```python
from build123d import *

# Parameters (mm, degrees)
BOSS_EXTRUDE1_DEPTH          = 21.6
SKETCH3_OUTSIDE_W            = 131.808
SKETCH3_OUTSIDE_H            = 138.238
SKETCH3_OUTSIDE_R            = 20.784609691
CUT_EXTRUDE1_DEPTH           = 21.6
CUT_EXTRUDE1_DRAFT           = -60
M24_TAPPED_HOLE1_D           = 21
M24_TAPPED_HOLE1_CSINK_D     = 24.05
M24_TAPPED_HOLE1_CSINK_ANGLE = 90


with BuildPart() as part:
    # Sketch1 → Boss-Extrude1 (new body)
    with BuildSketch(Plane.XY):
        Polygon((20.784609691, -12), (20.784609691, 12), (0, 24), (-20.784609691, 12), (-20.784609691, -12), (0, -24), align=None)
    extrude(amount=BOSS_EXTRUDE1_DEPTH)


with BuildPart() as cut_extrude1_tool:
    # Sketch3 outside → Cut-Extrude1 (with draft: the straight prism first)
    with BuildSketch(Plane.XY.offset(21.6)):
        Rectangle(SKETCH3_OUTSIDE_W, SKETCH3_OUTSIDE_H)
        Circle(SKETCH3_OUTSIDE_R, mode=Mode.SUBTRACT)
    extrude(amount=-CUT_EXTRUDE1_DEPTH)
    # Cut-Extrude1: the draft: its side faces are tilted about the plane it starts from
    cut_extrude1_sides = [cut_extrude1_tool.faces().sort_by_distance(p)[0] for p in [
        (0, -69.119, 10.8),
        (65.904, 0, 10.8),
        (0, 69.119, 10.8),
        (-65.904, 0, 10.8),
        (-20.784609691, 0, 10.8),
    ]]
    draft(cut_extrude1_sides, Plane.XY.offset(21.6), CUT_EXTRUDE1_DRAFT)


with BuildPart() as part_1:
    add(part.part)

    # Cut-Extrude1: cut by cut_extrude1_tool
    add(cut_extrude1_tool.part, mode=Mode.SUBTRACT)

    # M24 Tapped Hole1 (through all)
    with Locations(Plane.XY.offset(21.6)):
        with Locations((0, 0)):
            CounterSinkHole(M24_TAPPED_HOLE1_D / 2, M24_TAPPED_HOLE1_CSINK_D / 2, counter_sink_angle=M24_TAPPED_HOLE1_CSINK_ANGLE)


solid = part_1.part
```
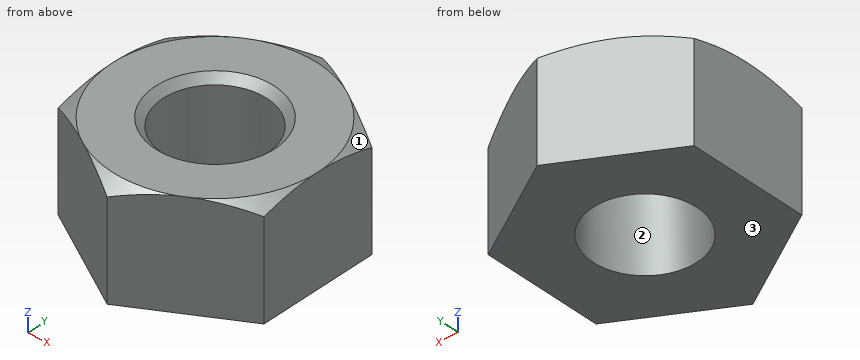
Here's how the part is built. I have some questions about the finished solid (model axes, mm). Face numbers are marked on the shaded views. Give positions to 0.01 mm unless a question says otherwise; leave off trailing zeros. Order: outer loops, then holes, each group sorted by start corner. A loop starts at its lowest first (then second) coordinate and runs counter-clockwise, first axis right, second up. Notation, with made-up numbers: (13.5, 17.5) - (28.5, 17.5) arc R14 ccw to (28.5, 31.5) - close; hole circle Ø8 at (53.5, 51.5). An arc over 180 degrees is marked (long way). Answer as a JSON object with one key per item and string values. Group by question number.
Item 1: If we section it at A-A on z = 2.5: Please give me the cut outline in (x, y).
Item 2: Please list where these lines run through material, in increasing order: probe 1 along Y at (x, z) = (0, 13.5); probe 2 along X at (y, z) = (0, 9.75); probe 3 along Y at (x, z) = (7, 9.75).
Item 3: If we mould it in two halves opening along X, with no side actions, what happens to the marked faces 1, 2 and 3? For each: pulls with the +X half, pulls with the -X half, needs draft (parallel to the pull), parting line crosses it, or undercut.
Item 4: For P1, Ø1, axis at y = -18.5, z = 12, coming from the +X side; P2, Ø8, axis at x = -8, z = 8.5, coming from the -Y side, each with a flat end and sliding along its axis, tell me the tip position at first contact or that it passes through.
Result set:
{
 "1": {"outline": "(-20.78, -12) - (0, -24) - (20.78, -12) - (20.78, 12) - (0, 24) - (-20.78, 12) - close; hole circle Ø21 at (0, 0)"},
 "2": {"probe 1": "-24 to -10.5, 10.5 to 24", "probe 2": "-20.78 to -10.5, 10.5 to 20.78", "probe 3": "-19.96 to -7.83, 7.83 to 19.96"},
 "3": {"face 1": "pulls with the +X half", "face 2": "undercut", "face 3": "needs draft"},
 "4": {"P1": "x = 10.39", "P2": "y = -21.69"}
}
